Study the drawing (mm; zero at the part's minimum x, y, z) and answer. A direction names the side the tool comes from. Round coordinates to 2 decimals unless told otherwise and drop trailing zeros. Write each loop counter-clockwise with the first axis right and the second up, starting at its lowest first coordinate (ties: lowest second). Pieces come first, ordered by that corner, then holes. Notation, with made-up numbers: (17, -11) -> (29, -11) arc R9 cw to (29, 6) -> close; hole circle Ø4 at (72, -10.5). An arc over 180 degrees is marked (long way). Return JSON: item names as keys, results as strings.
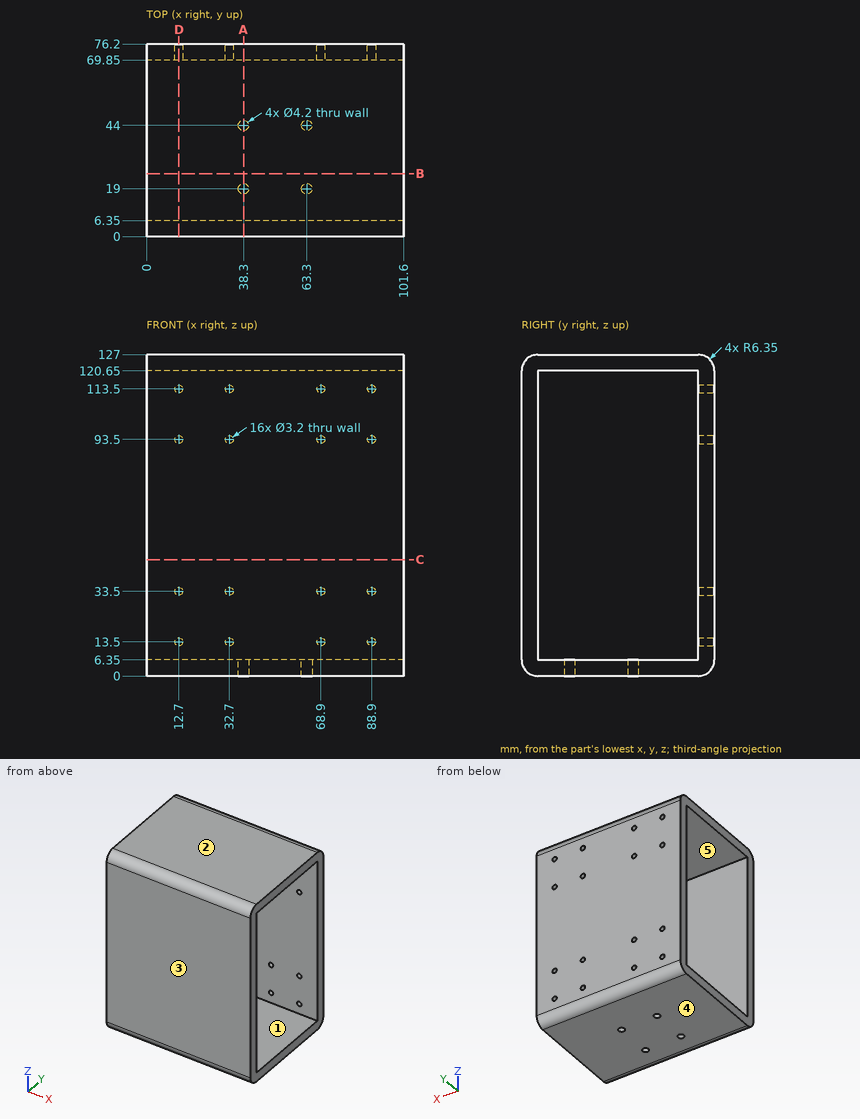
Item 1: Section A-A (x = 38.3) is taken. Give the vertices of the cut face in (y, z).
Worked answers:
{"outline": "(0, 6.35) arc R6.35 ccw to (6.35, 0) -> (16.9, 0) -> (16.9, 6.35) -> (6.35, 6.35) -> (6.35, 120.65) -> (69.85, 120.65) -> (69.85, 6.35) -> (46.1, 6.35) -> (46.1, 0) -> (69.85, 0) arc R6.35 ccw to (76.2, 6.35) -> (76.2, 120.65) arc R6.35 ccw to (69.85, 127) -> (6.35, 127) arc R6.35 ccw to (0, 120.65) -> close; (21.1, 0) -> (41.9, 0) -> (41.9, 6.35) -> (21.1, 6.35) -> close"}
Item 2: For a pull along Y with two mould halves and no side action, classify the marked faces 1, 2 and 3 as released by +Y, released by -Y, zero draft, split by the parting line, or undercut.
Worked answers:
{"face 1": "undercut", "face 2": "zero draft", "face 3": "released by -Y"}
Item 3: A tool of negligible diameter and unlimited length cuts with its end or side. For the marked faces 4 and 5, from which of +Z, -Z, +X, -X, +Y, -Y can it reach the whole face along a straight path? Write none if from no direction.
Worked answers:
{"face 4": "-Z, +X, -X, +Y, -Y", "face 5": "+X, -X"}
Item 4: Flat-ended cylindrical pins translate along their axes: pin 1 (2.5 mm diameter, centred on x = 68.9, z = 13.5, fed in from -Y); pin 2 (1.9 mm diameter, centred on x = 12.7, z = 33.5, fed in from +Y). Find the tip coordinate at first contact, or state that the pin passes through.
Worked answers:
{"pin 1": "stops at y = 0", "pin 2": "stops at y = 6.35"}
Item 5: Section D-D (x = 12.7) is taken. Give the vertices of the cut face in (y, z), then the cut area to 3 significant figures.
Worked answers:
{"outline": "(0, 6.35) arc R6.35 ccw to (6.35, 0) -> (69.85, 0) arc R6.35 ccw to (76.2, 6.35) -> (76.2, 11.9) -> (69.85, 11.9) -> (69.85, 6.35) -> (6.35, 6.35) -> (6.35, 120.65) -> (69.85, 120.65) -> (69.85, 115.1) -> (76.2, 115.1) -> (76.2, 120.65) arc R6.35 ccw to (69.85, 127) -> (6.35, 127) arc R6.35 ccw to (0, 120.65) -> close; (69.85, 15.1) -> (76.2, 15.1) -> (76.2, 31.9) -> (69.85, 31.9) -> close; (69.85, 35.1) -> (76.2, 35.1) -> (76.2, 91.9) -> (69.85, 91.9) -> close; (69.85, 95.1) -> (76.2, 95.1) -> (76.2, 111.9) -> (69.85, 111.9) -> close", "area": "2,300 mm2"}
Item 6: Section C-C (z = 46) is taken. Give the vertices of the cut face in (x, y), then the cut area to 3 significant figures.
Worked answers:
{"outline": "(0, 0) -> (101.6, 0) -> (101.6, 6.35) -> (0, 6.35) -> close; (0, 69.85) -> (101.6, 69.85) -> (101.6, 76.2) -> (0, 76.2) -> close", "area": "1,290 mm2"}
Item 7: Section B-B (y = 25) is taken. Give the vertices of the cut face in (x, z).
Worked answers:
{"outline": "(0, 0) -> (101.6, 0) -> (101.6, 6.35) -> (0, 6.35) -> close; (0, 120.65) -> (101.6, 120.65) -> (101.6, 127) -> (0, 127) -> close"}
Item 8: Straight lines are drawn through the part: L1, parallel to X at y = 72.75, z = 113.5; L2, parallel to Z at x = 11, y = 64.5; L3, parallel to Y at x = 8, z = 79.5. For each, find the intervals that lie inside material, in ascending order. Write a range as [from, to].
Worked answers:
{"L1": "x = [0, 11.1], [14.3, 31.1], [34.3, 67.3], [70.5, 87.3], [90.5, 101.6]", "L2": "z = [0, 6.35], [120.65, 127]", "L3": "y = [0, 6.35], [69.85, 76.2]"}
